Study the drawing (mm; zero at the part's minimum x, y, z) and answer. A direction names the side the tool comes from. Coordinates: 2 decimals unless noted, no trailing zeros. Order: outer loops, then holes, each group sorted by start corner. A loop starts at its lowest first (then second) coordinate and runs counter-clockwise, first axis right, second up. Notation, with made-up numbers: (8, 49.5) -> (55, 49.5) arc R17 cw to (55, 53.5) -> close; hole circle Ø4 at (20.5, 25.25). An arc over 180 degrees is marked (long way). Answer as CSV lines item,"result". Start each with the question number.
Item 1: Each of these flat-tipped pins is pushed along its axis until it touches: pin 1 Ø3 at (x, y) = (45.5, 20) entering from +Z; pin 2 Ø4 at (x, z) = (7, 2.5) entering from +Y; pin 3 Ø1.5 at (x, z) = (23.5, 13.5) entering from -Y; pin 4 Ø6.5 at (x, y) = (8, 20) entering from -Z. Where does it stop, or does it pass through?
Item 2: Section C-C (x = 32) is taken. Write down the section's boundary in (y, z), then the cut area to 3 significant figures.
Item 3: Section B-B (x = 8) is taken. Write down the section's boundary in (y, z), then the cut area to 3 significant figures.
Item 4: Section A-A (y = 20) is taken. Write down the section's boundary in (x, z).
Item 5: Straight lines are drawn through the part: L1, parallel to X at y = 20, z = 21.45; L2, parallel to Y at x = 8, z = 20.75; L3, parallel to X at y = 19.5, z = 20.5. For each, find the intervals that lie inside material, in ascending order.
Item 6: Which of the six approach directions +Z, -Z, +X, -X, +Y, -Y give full straight-line access (tool end or side, diameter ignored) to the marked faces 1 and 2?
Item 7: Section D-D (z = 2.5) is taken. Write down the section's boundary in (x, y).
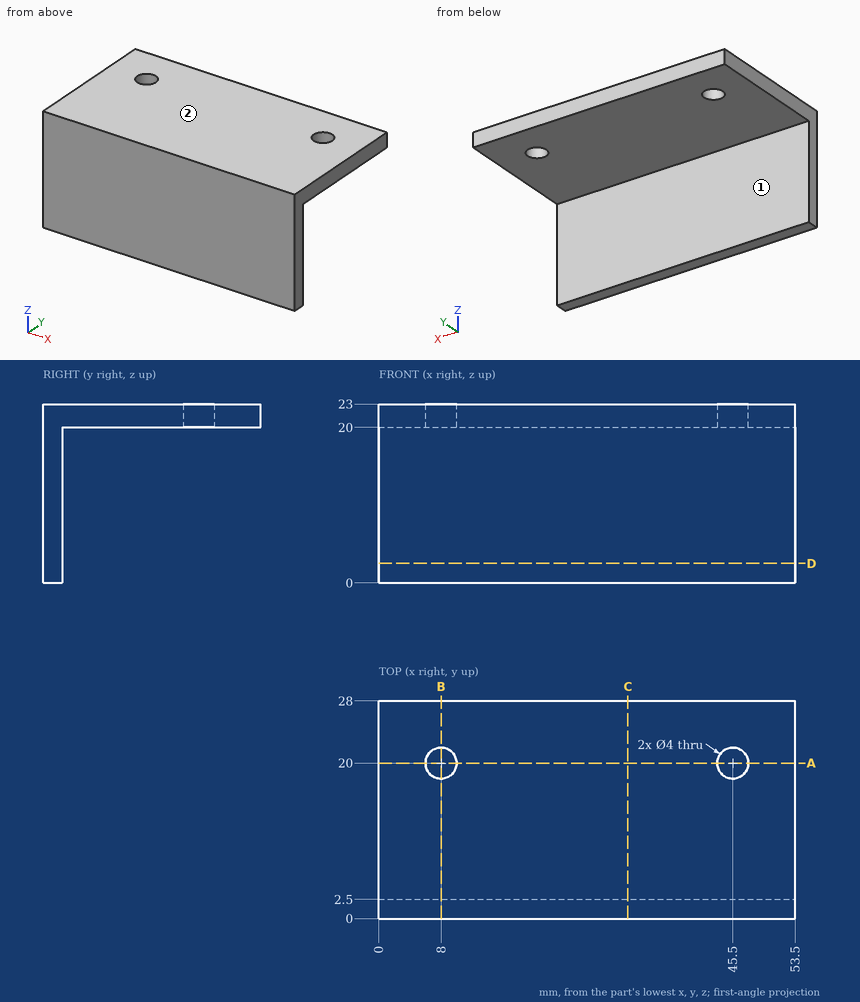
Checked values:
1,pin 1,"passes through"
1,pin 2,"stops at y = 2.5"
1,pin 3,"stops at y = 0"
1,pin 4,"stops at z = 20"
2,outline,"(0, 0) -> (2.5, 0) -> (2.5, 20) -> (28, 20) -> (28, 23) -> (0, 23) -> close"
2,area,"134 mm^2"
3,outline,"(0, 0) -> (2.5, 0) -> (2.5, 20) -> (18, 20) -> (18, 23) -> (0, 23) -> close; (22, 20) -> (28, 20) -> (28, 23) -> (22, 23) -> close"
3,area,"122 mm^2"
4,outline,"(0, 20) -> (6, 20) -> (6, 23) -> (0, 23) -> close; (10, 20) -> (43.5, 20) -> (43.5, 23) -> (10, 23) -> close; (47.5, 20) -> (53.5, 20) -> (53.5, 23) -> (47.5, 23) -> close"
5,L1,"x = 0 to 6, 10 to 43.5, 47.5 to 53.5"
5,L2,"y = 0 to 18, 22 to 28"
5,L3,"x = 0 to 6.06, 9.94 to 43.56, 47.44 to 53.5"
6,face 1,"-Z, +X, -X, +Y"
6,face 2,"+Z, +X, -X, +Y, -Y"
7,outline,"(0, 0) -> (53.5, 0) -> (53.5, 2.5) -> (0, 2.5) -> close"
